from build123d import *

# Parameters (mm, degrees)
BOSS_EXTRUDE1_DEPTH = 3
SKETCH2_W           = 40
SKETCH2_H           = 3
SKETCH2_W_2         = 45
BOSS_EXTRUDE2_DEPTH = 3
CUT_EXTRUDE1_DEPTH  = 3


with BuildPart() as part:
    # Sketch1 → Boss-Extrude1 (new body)
    with BuildSketch(Plane(origin=(0, 0, 0), x_dir=(1, 0, 0), z_dir=(0, 1, 0))):
        Polygon((-118.5, -30), (-118.5, -50), (121.5, -50), (121.5, -35), (124.5, -35), (124.5, -15), (121.5, -15), (121.5, 15), (124.5, 15), (124.5, 35), (121.5, 35), (121.5, 50), (-118.5, 50), (-118.5, 30), (-121.5, 30), (-121.5, 10), (-118.5, 10), (-118.5, -10), (-121.5, -10), (-121.5, -30), align=None)
    extrude(amount=BOSS_EXTRUDE1_DEPTH)

    # Sketch2 → Boss-Extrude2 (add)
    with BuildSketch(Plane(origin=(0, 0, -50), x_dir=(-1, 0, 0), z_dir=(0, 0, -1))):
        with Locations((-81.5, 1.5)):
            Rectangle(SKETCH2_W, SKETCH2_H)
        with Locations((1, 1.5)):
            Rectangle(SKETCH2_W_2, SKETCH2_H)
        with Locations((83.5, 1.5)):
            Rectangle(SKETCH2_W, SKETCH2_H)
    extrude(amount=BOSS_EXTRUDE2_DEPTH)

    # Sketch3 → Cut-Extrude1 (cut)
    with BuildSketch(Plane(origin=(0, 3, 0), x_dir=(1, 0, 0), z_dir=(0, 1, 0))):
        with BuildLine():
            Line((41.5, 25), (61.5, 25))
            ThreePointArc((61.5, 25), (68.571067812, 22.071067812), (71.5, 15))
            Line((71.5, 15), (71.5, -15))
            ThreePointArc((71.5, -15), (68.571067812, -22.071067812), (61.5, -25))
            Line((61.5, -25), (41.5, -25))
            ThreePointArc((41.5, -25), (34.428932188, -22.071067812), (31.5, -15))
            Line((31.5, -15), (31.5, 15))
            ThreePointArc((31.5, 15), (34.428932188, 22.071067812), (41.5, 25))
        make_face()
    extrude(amount=-CUT_EXTRUDE1_DEPTH, mode=Mode.SUBTRACT)


solid = part.part
The model under review builds one solid part; all positions refer to its coordinate system, in mm. A direction names the side the tool comes from. Give positions to 0.01 mm unless a question says otherwise; leave off trailing zeros. Order: outer loops, then holes, each group sorted by start corner. A loop starts at its lowest first (then second) coordinate and runs counter-clockwise, first axis right, second up. Notation, with made-up numbers: M 69,31.5 L 89,31.5 A14 cw 89,41.5 Z; hole C -27,71 d6. An arc over 180 degrees is marked long. One line per question, with ' | ' between items. Start each with the question number.
1) Wall thickness on L1, parallel to X at y = 1.3, z = -1.5; L2, parallel to Z at x = 45.5, y = 1.45; L3, parallel to X at y = 2.25, z = -47.5: over which ranges is each line inside the solid? List them lowest first. Write a range as from..to.
2) Consider section B-B, the plane x = -53.5. Give the boundary of the cut face in (y, z).
3) Consider section A-A, the plane z = 20. Give the boundary of the cut face in (x, y), then the cut area to 3 significant figures.
4) Consider section C-C, the plane z = -39. Give the boundary of the cut face in (x, y), then the cut area to 3 significant figures.
5) Clearance check with flat-ended pins moving along their axes: P1, Ø0.9, axis at x = 123, y = 2, coming from the -Z side; P2, Ø0.9, axis at x = -109, y = 2, coming from the -Z side; P3, Ø5, axis at x = 38.5, z = -30.5, coming from the -Y side; P4, Ø1.5, axis at y = 2, z = 41.5, coming from the -X side. State where each tip first meets the part, or that it passes through.
6) For faces 3 (the face through (68.49, 1.52, -22.15)), 4 (the face through (0, 0, -2)), list the 3-axis set-ups (+Z, -Z, +X, -X, +Y, -Y) from which the entire face can be reached by the end or side of a thin tool; tool diameter is ignored.
7) Mouldability with a two-part tool opening along X and no side actions: class faces 1 (the face through (34.51, 1.52, 22.15)), 2 (the face through (0, 3, -2)) as pulls with the +X half, pulls with the -X half, needs draft (parallel to the pull), parting line crosses it, or undercut.
Found:
1) L1: x = -118.5..31.5, 71.5..121.5 | L2: z = -50..-25, 25..50 | L3: x = -118.5..121.5
2) outline: M 0,-50 L 3,-50 L 3,50 L 0,50 Z
3) outline: M -121.5,0 L 32.84,0 L 32.84,3 L -121.5,3 Z; M 70.16,0 L 124.5,0 L 124.5,3 L 70.16,3 Z | area: 626 mm²
4) outline: M -118.5,0 L 121.5,0 L 121.5,3 L -118.5,3 Z | area: 720 mm²
5) P1: stops at z = -35 | P2: stops at z = -50 | P3: stops at y = 0 | P4: stops at x = -118.5
6) face 3: +Y, -Y | face 4: +Z, -Z, +X, -X, -Y
7) face 1: undercut | face 2: needs draft
